Work out the finished part from the listing and answer in its coordinate system (mm). A direction names the side the tool comes from. Coordinates: 2 decimals unless noted, no trailing zeros. Loops run counter-clockwise (first coordinate to the right, second up) from the corner with the lowest first, then second, coordinate; pieces in that order, holes last. Notation, with made-up numbers: M 65,-14 L 116,-14 A17 ccw 116,-1 Z; hole C 18.5,46 d6. An arc over 180 degrees is marked long. Write each question's results on one line, items separated by ' | '.
Autodesk Inventor part; units mm, degrees
ref_plane "YZ Plane" through (0, 0, 0) normal (1, 0, 0) x (0, 1, 0)
ref_plane "XZ Plane" through (0, 0, 0) normal (0, 1, 0) x (-1, 0, 0)
ref_plane "XY Plane" through (0, 0, 0) normal (0, 0, 1) x (1, 0, 0)
sketch "Sketch1" plane through (0, 0, 0) normal (0, 0, 1) x (1, 0, 0)
  line L0 (117.4905, 295.341) -> (6.3655, 295.341)
  line L1 (6.3655, 295.341) -> (6.3655, 257.241)
  line L2 (6.3655, 257.241) -> (117.4905, 257.241)
  line L3 (117.4905, 257.241) -> (117.4905, 295.341)
  line L4 (117.4905, 283.403) -> (6.3655, 283.403)
  line L5 (6.3655, 283.403) -> (6.3655, 281.773)
  line L6 (6.3655, 281.773) -> (117.4905, 281.773)
  line L7 (117.4905, 281.773) -> (117.4905, 283.403)
  line L8 (117.4905, 281.773) -> (117.4905, 283.403)
  line L9 (6.3655, 283.403) -> (11.128, 283.403)
  line L10 (11.128, 283.403) -> (11.128, 281.773)
  line L11 (11.128, 281.773) -> (6.3655, 281.773)
  line L12 (6.3655, 281.773) -> (6.3655, 283.403)
  line L13 (117.4905, 283.403) -> (114.3155, 283.403)
  line L14 (114.3155, 283.403) -> (114.3155, 281.773)
  line L15 (114.3155, 281.773) -> (117.4905, 281.773)
  line L16 (117.4905, 281.773) -> (117.4905, 283.403)
  point P0 (0, 0)
  dimension "d0" = 38.1
  dimension "d1" = 111.125
  dimension "d2" = 1.63
  dimension "d3" = 11.938
  dimension "d23" = 103.1875
  dimension "d24" = 3.175
extrude "Extrusion1" add sketch "Sketch1" along normal blind 3.175 contours L3 L4 L1 L0 | L3 L6 L14 L4 | L4 L10 L6 L1 | L3 L2 L1 L6
sketch "Sketch2" plane through (0, 0, 0) normal (0, 0, -1) x (-1, 0, 0)
  line L0 (-114.3155, 283.403) -> (-11.128, 283.403)
  line L1 (-26.2688, 289.3188) -> (-16.7438, 289.3188)
  line L2 (-16.7438, 289.3188) -> (-16.7438, 279.7938)
  line L3 (-16.7438, 279.7938) -> (-26.2688, 279.7938)
  line L4 (-26.2688, 279.7938) -> (-26.2688, 289.3188)
  line L5 (-96.4063, 289.4015) -> (-86.8813, 289.4015)
  line L6 (-86.8813, 289.4015) -> (-86.8813, 279.8838)
  line L7 (-86.8813, 279.8838) -> (-96.4063, 279.8838)
  line L8 (-96.4063, 279.8838) -> (-96.4063, 289.4015)
  line L9 (-6.3655, 257.241) -> (-117.4905, 257.241)
  line L10 (-6.3655, 295.341) -> (-6.3655, 257.241)
  line L11 (-77.4855, 257.241) -> (-49.5455, 257.241)
  line L12 (-49.5455, 257.241) -> (-49.5455, 267.401)
  line L13 (-49.5455, 267.401) -> (-77.4855, 267.401)
  line L14 (-77.4855, 267.401) -> (-77.4855, 257.241)
  line L15 (-117.4905, 257.241) -> (-117.4905, 295.341)
  line L16 (-117.4905, 295.341) -> (-6.3655, 295.341)
  line L17 (-53.9905, 295.341) -> (-41.2905, 295.341)
  line L18 (-41.2905, 295.341) -> (-41.2905, 292.801)
  line L19 (-41.2905, 292.801) -> (-53.9905, 292.801)
  line L20 (-53.9905, 292.801) -> (-53.9905, 295.341)
  point P0 (0, 0)
  point P1 (-117.4905, 283.403)
  point P2 (-6.3655, 283.403)
  dimension "d8" = 9.525
  dimension "d9" = 9.5177
  dimension "d10" = 9.525
  dimension "d11" = 9.525
  dimension "d13" = 5.9159
  dimension "d17" = 10.16
  dimension "d18" = 27.94
  dimension "d19" = 43.18
  dimension "d20" = 2.54
  dimension "d21" = 12.7
  dimension "d22" = 63.5
extrude "Extrusion2" cut sketch "Sketch2" against normal blind 3.175 contours L8 L5 L6 L0 | L0 L6 L7 L8 | L4 L1 L2 L0 | L0 L2 L3 L4 | L9 L14 L13 L12 | L18 L19 L20 L16
properties part number "RearBulkhead"
1) For a pull along X with two mould halves and no side action, classify faces 4 (the face through (57, 283.403, 2)), 5 (the face through (6.366, 277, 2)), 6 (the face through (97, 257.241, 2)) as released by +X, released by -X, zero draft, split by the parting line, or undercut.
Check result:
face 4: undercut | face 5: released by -X | face 6: zero draft
2) Find section D-D, the plane x = 95. Give the vertices of the cut face in (y, z) (1 decimal).
Check result:
outline: M 257.2,0 L 279.9,0 L 279.9,3.2 L 257.2,3.2 Z; M 289.4,0 L 295.3,0 L 295.3,3.2 L 289.4,3.2 Z
3) Straight lines are drawn through the part: probe 1 along X at (y, z) = (281, 0.2); probe 2 along Y at (x, z) = (27.5, 1.45); probe 3 along Y at (x, z) = (77, 2.55). For each, find the intervals that lie inside material, in ascending order. Write a range as [from, to].
Check result:
probe 1: [6.37, 16.74], [26.27, 86.88], [96.41, 117.49] | probe 2: [257.24, 281.77], [283.4, 295.34] | probe 3: [267.4, 281.77], [283.4, 295.34]
4) Which of the six approach directions +Z, -Z, +X, -X, +Y, -Y give full straight-line access (tool end or side, diameter ignored) to faces 1 (the face through (86, 295.341, 2)), 2 (the face through (92, 289.402, 2)), 3 (the face through (49.546, 262, 2))?
Check result:
face 1: +Z, -Z, +X, -X, +Y | face 2: +Z, -Z | face 3: +Z, -Z, -Y
5) Find section C-C, the plane y = 285. Give the vertices of the cut face in (x, z) (1 decimal), and give its area (3 significant figures).
Check result:
outline: M 6.4,0 L 16.7,0 L 16.7,3.2 L 6.4,3.2 Z; M 26.3,0 L 86.9,0 L 86.9,3.2 L 26.3,3.2 Z; M 96.4,0 L 117.5,0 L 117.5,3.2 L 96.4,3.2 Z | area: 292 mm^2
6) Find section A-A, the plane x = 76. Give the vertices of the cut face in (y, z) (3 decimals), and give its area (3 significant figures).
Check result:
outline: M 267.401,0 L 281.773,0 L 281.773,3.175 L 267.401,3.175 Z; M 283.403,0 L 295.341,0 L 295.341,3.175 L 283.403,3.175 Z | area: 83.5 mm^2
